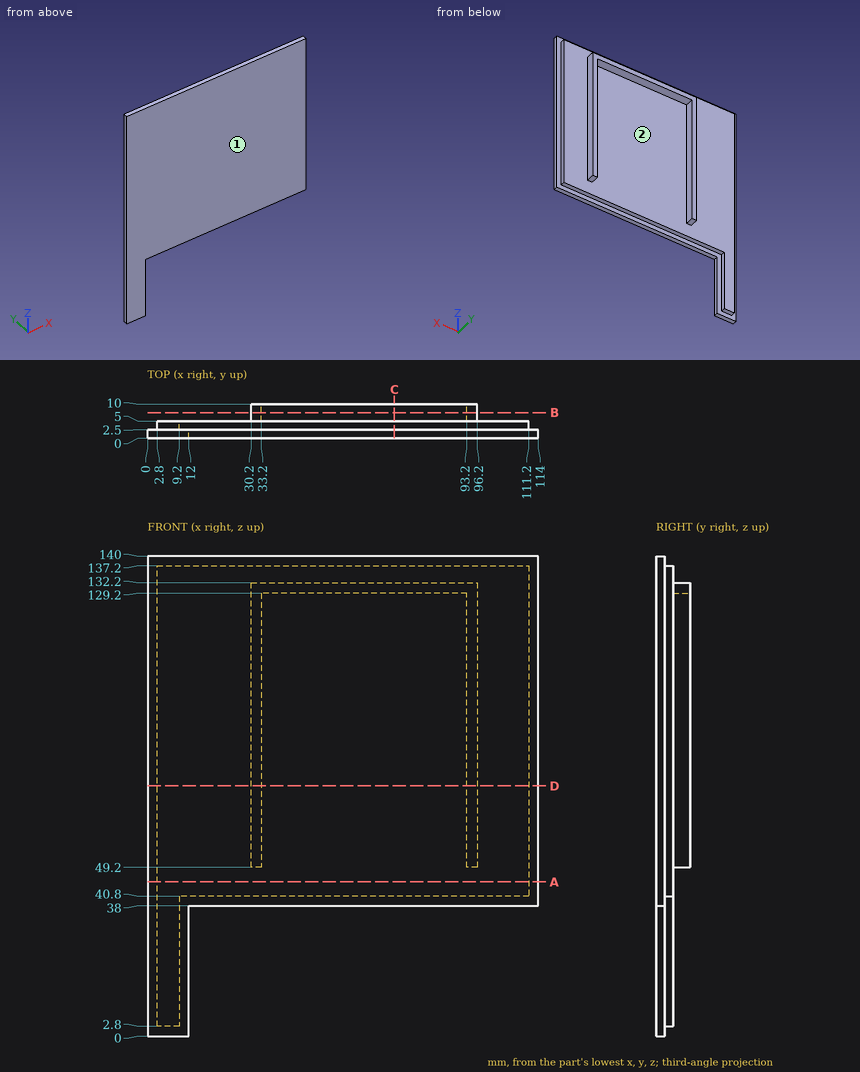
The drawing under review shows one solid part. Ordinate dimensions are in mm from its lowest x, y, z. Round coordinates to 2 decimals unless told otherwise and drop trailing zeros. Loops run counter-clockwise (first coordinate to the right, second up) from the corner with the lowest first, then second, coordinate; pieces in that order, holes last. Notation, with made-up numbers: (43.5, 78.5) - (84.5, 78.5) arc R4 ccw to (84.5, 83.5) - close; hole circle Ø3 at (49, 51.25). An arc over 180 degrees is marked (long way). One line per question, with ' | ' between items.
1. We need section D-D, the plane z = 73. State the section outline as (x, y) points, and give its area (3 significant figures).
Results are:
outline: (0, 0) - (114, 0) - (114, 2.5) - (111.2, 2.5) - (111.2, 5) - (96.2, 5) - (96.2, 10) - (93.2, 10) - (93.2, 5) - (33.2, 5) - (33.2, 10) - (30.2, 10) - (30.2, 5) - (2.8, 5) - (2.8, 2.5) - (0, 2.5) - close | area: 586 mm²
2. We need section A-A, the plane z = 45. State the section outline as (x, y) points, and give its area (3 significant figures).
Results are:
outline: (0, 0) - (114, 0) - (114, 2.5) - (111.2, 2.5) - (111.2, 5) - (2.8, 5) - (2.8, 2.5) - (0, 2.5) - close | area: 556 mm²
3. Clearance check with flat-ended pins moving along their axes: P1, Ø0.8, axis at y = 1.5, z = 24, coming from the +X side; P2, Ø3, axis at x = 68, y = 0.5, coming from the -Z side; P3, Ø1.5, axis at y = 7, z = 96.5, coming from the -X side. State where each tip first meets the part, or that it passes through.
Results are:
P1: stops at x = 12 | P2: stops at z = 38 | P3: stops at x = 30.2
4. We need section C-C, the plane x = 72. State the section outline as (y, z) points.
Results are:
outline: (0, 38) - (2.5, 38) - (2.5, 40.8) - (5, 40.8) - (5, 129.2) - (10, 129.2) - (10, 132.2) - (5, 132.2) - (5, 137.2) - (2.5, 137.2) - (2.5, 140) - (0, 140) - close
5. Draft analysis for pull direction X (two halves, no side actions). For the marked faces 1 and 2, state which applies: released by +X, released by -X, zero draft, split by the parting line, or undercut.
Results are:
face 1: zero draft | face 2: undercut
6. We need section B-B, the plane y = 7.5. State the section outline as (x, z) points, and give its area (3 significant figures).
Results are:
outline: (30.2, 49.2) - (33.2, 49.2) - (33.2, 129.2) - (93.2, 129.2) - (93.2, 49.2) - (96.2, 49.2) - (96.2, 132.2) - (30.2, 132.2) - close | area: 678 mm²
7. For L1, parallel to X at y = 8.75, z = 116; L2, parallel to Z at x = 94, y = 7; L3, parallel to X at y = 1.25, z = 10, list the stretches that pass through material, from the lowest coordinate up. Write a range as [from, to].
Results are:
L1: x = [30.2, 33.2], [93.2, 96.2] | L2: z = [49.2, 132.2] | L3: x = [0, 12]
